```python
from build123d import *

# Parameters (mm, degrees)
SKETCH1_W                                           = 10
SKETCH1_H                                           = 10
BOSS_EXTRUDE1_DEPTH                                 = 133
SKETCH3_W                                           = 1.8
SKETCH3_H                                           = 122
CUT_EXTRUDE1_DEPTH                                  = 5
FILLET1_R                                           = 0.9
SKETCH4_W                                           = 10
SKETCH4_H                                           = 10
BOSS_EXTRUDE3_DEPTH                                 = 15
CBORE_FOR_M3_HEX_SOCKET_HEAD_CAP_SCREW1_D           = 3.4
CBORE_FOR_M3_HEX_SOCKET_HEAD_CAP_SCREW1_CBORE_D     = 6.5
CBORE_FOR_M3_HEX_SOCKET_HEAD_CAP_SCREW1_CBORE_DEPTH = 3.4
F_1_0MM_DOWEL_HOLE1_D                               = 1
F_1_0MM_DOWEL_HOLE1_DEPTH                           = 8
F_1_0MM_DOWEL_HOLE1_TIP                             = 0.30043031


with BuildPart() as part:
    # Sketch1 → Boss-Extrude1 (new body)
    with BuildSketch(Plane(origin=(0, 0, 0), x_dir=(1, 0, 0), z_dir=(0, 1, 0))):
        Rectangle(SKETCH1_W, SKETCH1_H)
    extrude(amount=BOSS_EXTRUDE1_DEPTH)

    # Sketch3 → Cut-Extrude1 (cut)
    with BuildSketch(Plane(origin=(5, 0, 0), x_dir=(0, 0, -1), z_dir=(1, 0, 0))):
        with Locations((0, 72)):
            Rectangle(SKETCH3_W, SKETCH3_H)
    extrude(amount=-CUT_EXTRUDE1_DEPTH, mode=Mode.SUBTRACT)

    # Fillet1
    fillet1_edges = [part.edges().sort_by_distance(p)[0] for p in [
        (2.5, 11, 0.9),
        (2.5, 11, -0.9),
    ]]
    fillet(fillet1_edges, radius=FILLET1_R - 0.0001)  # a hair under: the kernel refuses the full size

    # Sketch4 → Boss-Extrude3 (add, symmetric)
    with BuildSketch(Plane(origin=(0, 0, 0), x_dir=(0, 0, -1), z_dir=(1, 0, 0))):
        with Locations((0, 5)):
            Rectangle(SKETCH4_W, SKETCH4_H)
    extrude(amount=BOSS_EXTRUDE3_DEPTH, both=True)

    # CBORE for M3 Hex Socket Head Cap Screw1 (through all)
    with Locations(Plane(origin=(10, 10, 0), x_dir=(0, 0, 1), z_dir=(0, 1, 0))):
        with Locations((0, 0)):
            cbore_for_m3_hex_socket_head_cap_screw1 = CounterBoreHole(CBORE_FOR_M3_HEX_SOCKET_HEAD_CAP_SCREW1_D / 2, CBORE_FOR_M3_HEX_SOCKET_HEAD_CAP_SCREW1_CBORE_D / 2, CBORE_FOR_M3_HEX_SOCKET_HEAD_CAP_SCREW1_CBORE_DEPTH)

    # Mirror1: CBORE for M3 Hex Socket Head Cap Screw1 across plane
    add(cbore_for_m3_hex_socket_head_cap_screw1.mirror(Plane(origin=(0, 0, 0), x_dir=(0, 0, 1), z_dir=(1, 0, 0))), mode=Mode.SUBTRACT)

    # Ø1.0mm Dowel Hole1
    with Locations(Plane(origin=(0, 0, 0), x_dir=(0, 0, -1), z_dir=(0, -1, 0))):
        with Locations((0, 0)):
            Hole(F_1_0MM_DOWEL_HOLE1_D / 2, depth=F_1_0MM_DOWEL_HOLE1_DEPTH)
            with Locations((0, 0, -(F_1_0MM_DOWEL_HOLE1_DEPTH + F_1_0MM_DOWEL_HOLE1_TIP / 2))):  # 118° drill point
                Cone(0, F_1_0MM_DOWEL_HOLE1_D / 2, F_1_0MM_DOWEL_HOLE1_TIP, mode=Mode.SUBTRACT)


solid = part.part
```
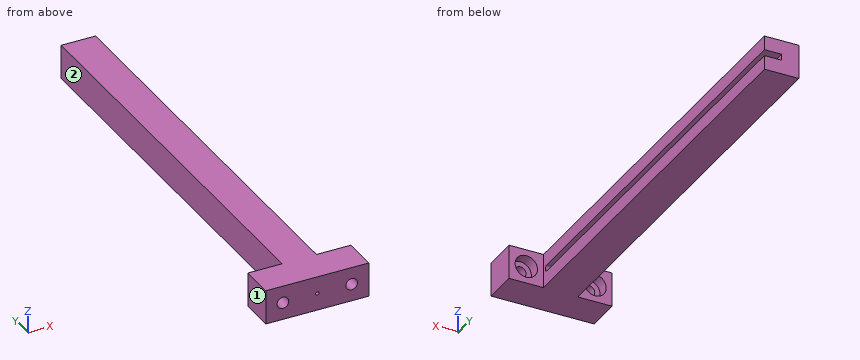
Source: CAD feature listing. Evaluate the final solid. Frame: model axes, mm. Face numbers are marked on the shaded views. A direction names the side the tool comes from. Give positions to 0.01 mm unless a question says otherwise; leave off trailing zeros. Write each loop counter-clockwise with the first axis right and the second up, starting at its lowest first coordinate (ties: lowest second). Pieces come first, ordered by that corner, then holes.
1. Material intervals for line 1 along X through (y, z) = (4.5, 0); line 2 along Z through (x, y) = (3.5, 45.5); line 3 along X through (y, z) = (78, 2.75), sorted ascending.
2. Section query A-A (y = 17). Return the cut outline in (x, z), then the cut area to 3 significant figures.
3. Access query for the marked faces 1 and 2. Directions: +Z, -Z, +X, -X, +Y, -Y. A direction counts if a zero-diameter tool reaches every point of the face in a straight line with its end or side. Return the directions, or none.
4. First-contact query: pin 1 (5 mm diameter, centred on x = -10, z = 0.5, fed in from +Y); pin 2 (1.4 mm diameter, centred on y = 82, z = 0, fed in from +X); pin 3 (5 mm diameter, centred on y = 65, z = -2, fed in from -X). Flat tips, straight axial feed; report the tip coordinate or a pass-through.
5. Section query B-B (x = -10). Return the cut outline in (y, z), then the cut area to 3 significant figures.
Output values:
1. line 1: x = -15 to -11.7, -8.3 to -0.5, 0.5 to 8.3, 11.7 to 15
1. line 2: z = -5 to -0.9, 0.9 to 5
1. line 3: x = -5 to 5
2. outline: (-5, -5) - (5, -5) - (5, -0.9) - (0, -0.9) - (0, 0.9) - (5, 0.9) - (5, 5) - (-5, 5) - close
2. area: 91.0 mm2
3. face 1: +Z, -Z, -X, +Y, -Y
3. face 2: +Z, -Z, -X, +Y
4. pin 1: stops at y = 6.6
4. pin 2: stops at x = 0
4. pin 3: stops at x = -5
5. outline: (0, -5) - (10, -5) - (10, -3.25) - (6.6, -3.25) - (6.6, -1.7) - (0, -1.7) - close; (0, 1.7) - (6.6, 1.7) - (6.6, 3.25) - (10, 3.25) - (10, 5) - (0, 5) - close
5. area: 55.5 mm2
